Geometry check sheet. Reference: the model listing, model coordinates, mm. Face numbers are marked on the shaded views. A direction names the side the tool comes from. Coordinates: 2 decimals unless noted, no trailing zeros. Write each loop counter-clockwise with the first axis right and the second up, starting at its lowest first coordinate (ties: lowest second). Pieces come first, ordered by that corner, then holes. Notation, with made-up numbers: (24, 64.25) -> (56, 64.25) arc R28 ccw to (56, 89.25) -> close; hole circle Ø3 at (39, 73.25). An arc over 180 degrees is marked (long way). Answer in a Markdown table with one row per item. Add a question column.
1. Scan lines: L1, parallel to Y at x = 89.5, z = 27; L2, parallel to Z at x = 3.5, y = 11.5; L3, parallel to X at y = -16.5, z = -36. Record each from-to range of solid material in increasing order. Write a range as from..to.
2. Depth check by flat-ended pin: P1, Ø5, axis at x = 111.5, y = 60, coming from the -Z side; P2, Ø12.5, axis at y = 29, z = 17, coming from the -X side; P3, Ø10, axis at x = 56, y = 50, coming from the +Z side. Enter the tip coordinate at first touch or a pass-through.
3. Cross-section at D-D on z = -17.5. Record the cut outline in (x, y).
4. Set-up check for the marked faces 1, 2 and 3: record each of +Z, -Z, +X, -X, +Y, -Y from which the full face is reachable in a straight line by a thin tool's end or side.
5. Cross-section at C-C on y = 60. Record the cut outline in (x, z), and give its area (4 significant figures).
6. Mould release check, pull along Y, two halves, no side actions. Record for the marked faces 4, 5 and 6: pulls with the +Y half, pulls with the -Y half, needs draft (parallel to the pull), parting line crosses it, or undercut.
7. Cross-section at A-A on z = 15. Record the cut outline in (x, y).
8. Cross-section at B-B on x = 87.5. Record the cut outline in (y, z).
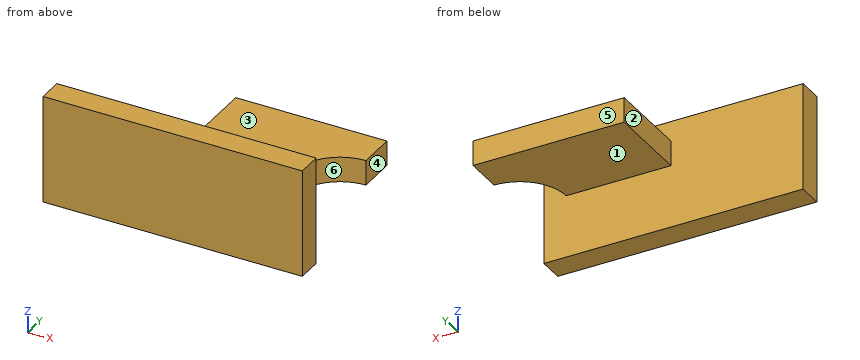
```python
from build123d import *

# Parameters (mm, degrees)
F0_W     = 263.6432349682
F0_H     = 109.4194687903
F0_W_2   = 227.0261347294
F0_H_2   = 80.9316635132
F1_DEPTH = 25.4
F3_DEPTH = 25.4


with BuildPart() as f1:
    # F0 (on Front) → F1 (new body)
    with BuildSketch(Plane.XZ):
        with Locations((-2.4411380291, -8.943548426)):
            Rectangle(F0_W, F0_H)
        with Locations((-3.0514225364, -5.458008498)):
            Rectangle(F0_W_2, F0_H_2, mode=Mode.SUBTRACT)
        with Locations((-3.0514225364, -5.458008498)):
            Rectangle(F0_W_2, F0_H_2)
    extrude(amount=F1_DEPTH)

    # F2 (on Top) → F3 (join)
    with BuildSketch(Plane.XY):
        with BuildLine():
            Line((0, 85.7104361057), (0, 0))
            Line((0, 0), (106.6103050285, 0))
            ThreePointArc((106.6103050285, 0), (120.414287269, 33.3257611396), (153.7400484085, 47.12974338))
            Line((153.7400484085, 47.12974338), (153.7400484085, 85.7104361057))
            Line((153.7400484085, 85.7104361057), (0, 85.7104361057))
        make_face()
    extrude(amount=F3_DEPTH)


solid = f1.part
```
Results found:
| question | item | result |
|---|---|---|
| 1 | L1 | y = -25.4..0 |
| 1 | L2 | z = 0..25.4 |
| 1 | L3 | x = -134.26..129.38 |
| 2 | P1 | stops at z = 0 |
| 2 | P2 | stops at x = 0 |
| 2 | P3 | stops at z = 25.4 |
| 3 | outline | (-134.26, -25.4) -> (129.38, -25.4) -> (129.38, 0) -> (-134.26, 0) -> close |
| 4 | face 1 | -Z, +X, -X, +Y |
| 4 | face 2 | +Z, -Z, -X, +Y |
| 4 | face 3 | +Z, +X, -X, +Y |
| 5 | outline | (0, 0) -> (153.74, 0) -> (153.74, 25.4) -> (0, 25.4) -> close |
| 5 | area | 3,905 mm^2 |
| 6 | face 4 | needs draft |
| 6 | face 5 | pulls with the +Y half |
| 6 | face 6 | undercut |
| 7 | outline | (-134.26, -25.4) -> (129.38, -25.4) -> (129.38, 0) -> (106.61, 0) arc R47.13 cw to (153.74, 47.13) -> (153.74, 85.71) -> (0, 85.71) -> (0, 0) -> (-134.26, 0) -> close |
| 8 | outline | (-25.4, -63.65) -> (0, -63.65) -> (0, 0) -> (85.71, 0) -> (85.71, 25.4) -> (0, 25.4) -> (0, 45.77) -> (-25.4, 45.77) -> close |
